Work out the finished part from the listing and answer in its coordinate system (mm). Face numbers are marked on the shaded views. A direction names the side the tool comes from. Round coordinates to 2 decimals unless told otherwise and drop trailing zeros. Loops run counter-clockwise (first coordinate to the right, second up) from the corner with the lowest first, then second, coordinate; pieces in that order, holes last. Notation, with made-up numbers: M 80.5,45.25 L 90.5,45.25 A16 cw 90.5,69.25 Z; hole C 19.5,-38 d7. An arc over 180 degrees is marked long. One line per item, written item: value.
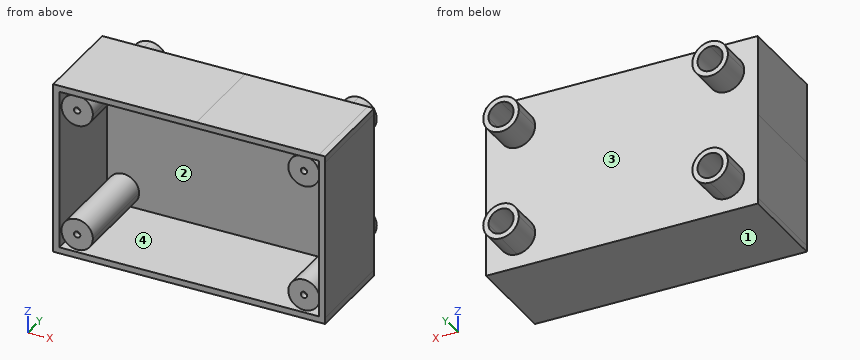
```python
from build123d import *

# Parameters (mm, degrees)
F0_W     = 210
F0_H     = 130
F1_DEPTH = 2
F2_DEPTH = 76.2
F4_DEPTH = 25.4
F5_R     = 2.54
F6_DEPTH = 72
F7_DEPTH = 66.929


with BuildPart() as f1:
    # F0 (on Front) → F1 (new body)
    with BuildSketch(Plane.XZ):
        with Locations((-6.0398806084, -4.6014347222)):
            Rectangle(F0_W, F0_H)
    extrude(amount=F1_DEPTH)

    # F0 (on Front) → F2 (join)
    with BuildSketch(Plane.XZ):
        Polygon((-0.235864222, 65.4023652778), (-111.0638493299, 65.4023652778), (-116.0436806083, 65.4023652778), (-116.0436806083, 60.398529828), (-116.0436806083, -4.06776e-05), (-116.0436806084, -69.6014285846), (-116.0436806084, -74.6014347222), (-111.0398806084, -74.6014347222), (98.9601193916, -74.6014347222), (103.9639193853, -74.6014347222), (103.9639193853, -69.6011838004), (103.9639193916, 60.3988544052), (103.9639193916, 65.3985652778), (98.9361506701, 65.3985652778), align=None)
        with Locations((-6.0398806084, -4.6014347222)):
            Rectangle(F0_W, F0_H, mode=Mode.SUBTRACT)
    extrude(amount=F2_DEPTH)

    # F3 (on face) → F4 (join)
    with BuildSketch(Plane(origin=(0, 0, 0), x_dir=(-1, 0, 0), z_dir=(0, 1, 0))):
        with BuildLine():
            ThreePointArc((-92.9588075555, 39.9985652778), (-78.5639193916, 25.6036771139), (-64.1690312277, 39.9985652778))
            ThreePointArc((-64.1690312277, 39.9985652778), (-68.3851963565, 50.1772883129), (-78.5639193916, 54.3934534417))
            Line((-78.5639193916, 54.3934534417), (-78.5639193916, 50.1585652778))
            ThreePointArc((-78.5639193916, 50.1585652778), (-71.3797144948, 47.1827701747), (-68.4039193916, 39.9985652778))
            ThreePointArc((-68.4039193916, 39.9985652778), (-78.5639193916, 29.8385652778), (-88.7239193916, 39.9985652778))
            Line((-88.7239193916, 39.9985652778), (-92.9588075555, 39.9985652778))
        make_face()
        with BuildLine():
            Line((-78.5639193916, 50.1585652778), (-78.5639193916, 54.3934534417))
            ThreePointArc((-78.5639193916, 54.3934534417), (-88.7426424267, 50.1772883129), (-92.9588075555, 39.9985652778))
            Line((-92.9588075555, 39.9985652778), (-88.7239193916, 39.9985652778))
            ThreePointArc((-88.7239193916, 39.9985652778), (-85.7481242885, 47.1827701747), (-78.5639193916, 50.1585652778))
        make_face()
        with BuildLine():
            ThreePointArc((-64.1690312214, -49.2014347222), (-78.5639193853, -34.8065465583), (-92.9588075492, -49.2014347222))
            Line((-92.9588075492, -49.2014347222), (-88.7239193853, -49.2014347222))
            ThreePointArc((-88.7239193853, -49.2014347222), (-78.5639193853, -39.0414347222), (-68.4039193853, -49.2014347222))
            ThreePointArc((-68.4039193853, -49.2014347222), (-71.3797144885, -56.385639619), (-78.5639193853, -59.3614347222))
            Line((-78.5639193853, -59.3614347222), (-78.5639193853, -63.5963228861))
            ThreePointArc((-78.5639193853, -63.5963228861), (-68.3851963502, -59.3801577573), (-64.1690312214, -49.2014347222))
        make_face()
        with BuildLine():
            Line((-88.7239193853, -49.2014347222), (-92.9588075492, -49.2014347222))
            ThreePointArc((-92.9588075492, -49.2014347222), (-88.7426424204, -59.3801577573), (-78.5639193853, -63.5963228861))
            Line((-78.5639193853, -63.5963228861), (-78.5639193853, -59.3614347222))
            ThreePointArc((-78.5639193853, -59.3614347222), (-85.7481242822, -56.385639619), (-88.7239193853, -49.2014347222))
        make_face()
        with BuildLine():
            ThreePointArc((105.0385687722, 40.0023652778), (100.8224036434, 50.1810883129), (90.6436806083, 54.3972534417))
            Line((90.6436806083, 54.3972534417), (90.6436806083, 50.1623652778))
            ThreePointArc((90.6436806083, 50.1623652778), (97.8278855051, 47.1865701747), (100.8036806083, 40.0023652778))
            Line((100.8036806083, 40.0023652778), (105.0385687722, 40.0023652778))
        make_face()
        with BuildLine():
            Line((90.6436806083, 50.1623652778), (90.6436806083, 54.3972534417))
            ThreePointArc((90.6436806083, 54.3972534417), (80.4649575731, 29.8236422427), (105.0385687722, 40.0023652778))
            Line((105.0385687722, 40.0023652778), (100.8036806083, 40.0023652778))
            ThreePointArc((100.8036806083, 40.0023652778), (83.4594757114, 32.818160381), (90.6436806083, 50.1623652778))
        make_face()
        with BuildLine():
            ThreePointArc((105.0385687723, -49.2014347222), (80.4649575733, -39.0227116871), (90.6436806084, -63.5963228861))
            Line((90.6436806084, -63.5963228861), (90.6436806084, -59.3614347222))
            ThreePointArc((90.6436806084, -59.3614347222), (83.4594757115, -42.0172298253), (100.8036806084, -49.2014347222))
            Line((100.8036806084, -49.2014347222), (105.0385687723, -49.2014347222))
        make_face()
        with BuildLine():
            Line((90.6436806084, -59.3614347222), (90.6436806084, -63.5963228861))
            ThreePointArc((90.6436806084, -63.5963228861), (100.8224036435, -59.3801577573), (105.0385687723, -49.2014347222))
            Line((105.0385687723, -49.2014347222), (100.8036806084, -49.2014347222))
            ThreePointArc((100.8036806084, -49.2014347222), (97.8278855052, -56.385639619), (90.6436806084, -59.3614347222))
        make_face()
    extrude(amount=F4_DEPTH)

    # F5 (on face) → F6 (join)
    with BuildSketch(Plane.XZ.offset(2)):
        with BuildLine():
            ThreePointArc((98.4618922379, -56.3934347222), (76.7816361169, -47.4131786011), (85.7618922379, -69.0934347222))
            ThreePointArc((85.7618922379, -69.0934347222), (94.742148359, -65.3736908433), (98.4618922379, -56.3934347222))
        make_face()
        with Locations((85.7618922379, -56.3934347222)):
            Circle(F5_R, mode=Mode.SUBTRACT)
        with BuildLine():
            ThreePointArc((-110.5318806084, -56.3934347222), (-106.8121367295, -65.3736908433), (-97.8318806084, -69.0934347222))
            ThreePointArc((-97.8318806084, -69.0934347222), (-88.8516244873, -65.3736908433), (-85.1318806084, -56.3934347222))
            ThreePointArc((-85.1318806084, -56.3934347222), (-97.8318806084, -43.6934347222), (-110.5318806084, -56.3934347222))
        make_face()
        with Locations((-97.8318806084, -56.3934347222)):
            Circle(F5_R, mode=Mode.SUBTRACT)
        with BuildLine():
            ThreePointArc((-97.8318806084, 59.8905652778), (-106.8121367295, 56.1708213989), (-110.5318806084, 47.1905652778))
            ThreePointArc((-110.5318806084, 47.1905652778), (-97.8318806084, 34.4905652778), (-85.1318806084, 47.1905652778))
            ThreePointArc((-85.1318806084, 47.1905652778), (-88.8516244873, 56.1708213989), (-97.8318806084, 59.8905652778))
        make_face()
        with Locations((-97.8318806084, 47.1905652778)):
            Circle(F5_R, mode=Mode.SUBTRACT)
        with BuildLine():
            ThreePointArc((85.7521193916, 59.8905652778), (76.7718632705, 38.2103091567), (98.4521193916, 47.1905652778))
            ThreePointArc((98.4521193916, 47.1905652778), (94.7323755127, 56.1708213989), (85.7521193916, 59.8905652778))
        make_face()
        with Locations((85.7521193916, 47.1905652778)):
            Circle(F5_R, mode=Mode.SUBTRACT)
    extrude(amount=F6_DEPTH)

    # F5 (on face) → F7 (join)
    with BuildSketch(Plane.XZ.offset(2)):
        with Locations((-97.8318806084, -56.3934347222)):
            Circle(F5_R)
        with Locations((85.7618922379, -56.3934347222)):
            Circle(F5_R)
        with Locations((-97.8318806084, 47.1905652778)):
            Circle(F5_R)
        with Locations((85.7521193916, 47.1905652778)):
            Circle(F5_R)
    extrude(amount=F7_DEPTH)


solid = f1.part
```
1) Each of these flat-tipped pins is pushed along its axis until it touches: pin 1 (5 mm diameter, centred on x = 36.5, z = -11.5, fed in from +Y); pin 2 (22.5 mm diameter, centred on x = 75.5, z = 40.5, fed in from +Y); pin 3 (16.5 mm diameter, centred on x = -90.64, z = 40, fed in from -Y); pin 4 (5 mm diameter, centred on x = -85, y = 14, fed in from +Z). Where does it stop, or does it pass through?
Check values:
pin 1: y = 0
pin 2: y = 25.4
pin 3: y = -74
pin 4: z = 54.05
2) Find section C-C (x = -47.5). Give the vertices of the cut face in (y, z), then the cut area to 3 significant figures.
Check values:
outline: M -76.2,-74.6 L 0,-74.6 L 0,65.4 L -76.2,65.4 L -76.2,60.4 L -2,60.4 L -2,-69.6 L -76.2,-69.6 Z
area: 1,020 mm2
3) For the marked faces 3 and 4, determine the directions among +Z, -Z, +X, -X, +Y, -Y from which every point of the face is accessible in a straight line to the end or side of a thin tool.
Check values:
face 3: +Y
face 4: -Y
4) Find section A-A (y = -39). Give the vertices of the cut face in (x, z), then the cut area to 3 significant figures.
Check values:
outline: M -116.04,-74.6 L 103.96,-74.6 L 103.96,65.4 L 98.94,65.4 L -0.24,65.4 L -116.04,65.4 Z; C -97.83,-56.39 d25.4; C -97.83,47.19 d25.4; C 85.75,47.19 d25.4; C 85.76,-56.39 d25.4; hole M -111.04,-69.6 L 98.96,-69.6 L 98.96,60.4 L -111.04,60.4 Z
area: 5,530 mm2
5) Find the intervals of material crossed by probe 1 along Z at (x, y) = (-98, -28); probe 2 along X at (y, z) = (-41.5, -55.5); probe 3 along Z at (x, y) = (0, -50.5), in increasing order. Write a range as from..to.
Check values:
probe 1: -74.6..-69.6, -69.09..-43.69, 34.49..59.89, 60.4..65.4
probe 2: -116.04..-111.04, -110.5..-85.16, 73.09..98.43, 98.96..103.96
probe 3: -74.6..-69.6, 60.4..65.4
6) The mould has two halves that part along Z. Classify the marked faces 1 and 2: +Z half, -Z half, draft (parallel to the pull), parting line (faces both ways), or undercut.
Check values:
face 1: -Z half
face 2: undercut
7) Find section D-D (z = 14). Give the vertices of the cut face in (x, y), then the cut area to 3 significant figures.
Check values:
outline: M -116.04,-76.2 L -111.04,-76.2 L -111.04,-2 L 98.96,-2 L 98.96,-76.2 L 103.96,-76.2 L 103.96,0 L -116.04,0 Z
area: 1,180 mm2
8) Find section B-B (y = 16.5). Give the vertices of the cut face in (x, z), then the cut area to 3 significant figures.
Check values:
outline: C -90.64,-49.2 d28.79; C -90.64,40 d28.79; C 78.56,-49.2 d28.79; C 78.56,40 d28.79; hole C -90.64,-49.2 d20.32; hole C -90.64,40 d20.32; hole C 78.56,-49.2 d20.32; hole C 78.56,40 d20.32
area: 1,310 mm2
